Source: CAD feature listing. Evaluate the final solid. Frame: model axes, mm. A direction names the side the tool comes from. Give positions to 0.01 mm unless a question says otherwise; leave off trailing zeros. Write each loop counter-clockwise with the first axis right and the second up, starting at its lowest first coordinate (ties: lowest second). Pieces come first, ordered by that corner, then holes. Notation, with made-up numbers: M 12.25,60 L 47.25,60 A15 cw 47.25,79 Z; hole C 39.25,86 d11. An arc over 180 degrees is marked long. Answer as a JSON object with one key per item and string values. Group by question number.
Autodesk Inventor part; units mm, degrees
ref_plane "YZ Plane" through (0, 0, 0) normal (1, 0, 0) x (0, 1, 0)
ref_plane "XZ Plane" through (0, 0, 0) normal (0, 1, 0) x (-1, 0, 0)
ref_plane "XY Plane" through (0, 0, 0) normal (0, 0, 1) x (1, 0, 0)
sketch "Sketch1" plane through (0, 0, 0) normal (0, 0, 1) x (1, 0, 0)
  line L0 (-51.8104, 0) -> (51.8104, 0) construction
  line L1 (0, -35.1144) -> (0, 36.3819) construction
  line L2 (0, 0) -> (26.1682, 26.1682) construction
  line L3 (0, 0) -> (37.0074, 0) construction
  line L4 (16.8, 24.9006) -> (16.8, 21.2406)
  line L5 (16.8, 21.2406) -> (19.0203, 19.0203)
  line L6 (16.8, 24.9006) -> (0, 24.9006)
  line L7 (24.9006, 16.8) -> (21.2406, 16.8)
  line L8 (21.2406, 16.8) -> (19.0203, 19.0203)
  line L9 (24.9006, 16.8) -> (24.9006, 0)
  line L10 (0, 0) -> (-37.0074, 0) construction
  line L11 (-16.8, 24.9006) -> (-16.8, 21.2406)
  line L12 (-16.8, 21.2406) -> (-19.0203, 19.0203)
  line L13 (-16.8, 24.9006) -> (0, 24.9006)
  line L14 (-24.9006, 16.8) -> (-24.9006, 0)
  line L15 (-24.9006, 16.8) -> (-21.2406, 16.8)
  line L16 (-21.2406, 16.8) -> (-19.0203, 19.0203)
  line L17 (16.8, -24.9006) -> (16.8, -21.2406)
  line L18 (16.8, -21.2406) -> (19.0203, -19.0203)
  line L19 (16.8, -24.9006) -> (0, -24.9006)
  line L20 (24.9006, -16.8) -> (24.9006, 0)
  line L21 (24.9006, -16.8) -> (21.2406, -16.8)
  line L22 (21.2406, -16.8) -> (19.0203, -19.0203)
  line L23 (-16.8, -24.9006) -> (-16.8, -21.2406)
  line L24 (-16.8, -21.2406) -> (-19.0203, -19.0203)
  line L25 (-16.8, -24.9006) -> (0, -24.9006)
  line L26 (-24.9006, -16.8) -> (-24.9006, 0)
  line L27 (-24.9006, -16.8) -> (-21.2406, -16.8)
  line L28 (-21.2406, -16.8) -> (-19.0203, -19.0203)
  line L29 (-16.8, -16.8) -> (16.8, 16.8) construction
  line L30 (17.4242, -17.4242) -> (-16.0391, 16.0391) construction
  line L31 (-16.8, -15) -> (16.8, -15)
  line L32 (16.8, -15) -> (16.8, 15)
  line L33 (16.8, 15) -> (-16.8, 15)
  line L34 (-16.8, 15) -> (-16.8, -15)
  line L35 (-16.8, -15) -> (16.8, 15) construction
  line L36 (16.8, -15) -> (-16.8, 15) construction
  dimension "d0" = 45
  dimension "d1" = 3.14
  dimension "d2" = 3.66
  dimension "d4" = 16.8
  dimension "d16" = 33.6
  dimension "d17" = 30
extrude "Extrusion1" add sketch "Sketch1" along normal blind 8
sketch "Sketch2" plane through (-16.8, 24.9006, 0) normal (0, 1, 0) x (1, 0, 0)
  line L0 (-8.1006, 0) -> (-4.4406, 0) construction
  line L1 (-8.1006, 0) -> (-8.1006, -8) construction
  line L2 (-4.4406, -8) -> (-8.1006, -8) construction
  line L3 (-4.4406, 0) -> (-4.4406, -8) construction
  line L4 (-4.4406, 0) -> (0, 0) construction
  line L5 (-4.4406, 0) -> (-4.4406, -8) construction
  line L6 (0, -8) -> (-4.4406, -8) construction
  line L7 (0, 0) -> (0, -8) construction
  line L8 (0, 0) -> (33.6, 0) construction
  line L9 (0, 0) -> (0, -8) construction
  line L10 (33.6, -8) -> (0, -8) construction
  line L11 (33.6, 0) -> (33.6, -8) construction
  line L12 (33.6, 0) -> (38.0406, 0) construction
  line L13 (33.6, 0) -> (33.6, -8) construction
  line L14 (38.0406, -8) -> (33.6, -8) construction
  line L15 (38.0406, 0) -> (38.0406, -8) construction
  line L16 (38.0406, 0) -> (41.7006, 0) construction
  line L17 (38.0406, 0) -> (38.0406, -8) construction
  line L18 (41.7006, -8) -> (38.0406, -8) construction
  line L19 (41.7006, 0) -> (41.7006, -8) construction
  line L20 (-0.9933, -0.6346) -> (2.8461, 5.7642) construction
  ellipse E0 centre (4.1754, 7.1215) end of major axis (2.3333, 6.6563) minor radius 1.8997 (5.4585, 5.7204) -> (2.8461, 5.7642) ccw construction
  line L21 (5.4585, 5.7204) -> (9.3415, -1.2728) construction
  line L22 (9.3415, -1.2728) -> (8.4179, -1.2574) construction
  line L23 (8.4179, -1.2574) -> (4.8304, 5.2036) construction
  ellipse E1 centre (5.2675, 5.4463) end of major axis (4.7828, 5.3239) minor radius 0.4999 (4.9945, 5.8651) -> (4.8304, 5.2036) ccw construction
  ellipse E2 centre (4.1754, 7.1215) end of major axis (2.7211, 6.7542) minor radius 1.4998 (4.9945, 5.8651) -> (3.3146, 5.8932) ccw construction
  ellipse E3 centre (3.0277, 5.4838) end of major axis (3.5125, 5.6062) minor radius 0.4999 (3.4564, 5.2266) -> (3.3146, 5.8932) ccw construction
  line L24 (3.4564, 5.2266) -> (-0.3461, -1.1107) construction
  ellipse E4 centre (-1.5262, -2.0366) end of major axis (-0.0719, -1.6693) minor radius 1.4998 (-0.9933, -0.6346) -> (-0.3461, -1.1107) ccw construction
  circle A0 centre (-2.1474, -2.1474) radius 1.7
  line L25 (-4.4406, 0) -> (0, 0) construction
  line L26 (0, 0) -> (-3.5302, -3.5302) construction
  line L27 (0, 0) -> (4.9925, 0) construction
  line L28 (0, 0) -> (2, 0)
  line L29 (0, 0) -> (-1.7777, 0)
  line L30 (-1.7777, 0) -> (-2.227, -0.4493)
  line L31 (0, 0) -> (0, -3.2892)
  line L32 (0, -3.2892) -> (-0.8879, -3.2892)
  point P0 (16.8, 0)
  dimension "d8" = 3.4
  dimension "d9" = 135
extrude "Extrusion2" cut sketch "Sketch2" against normal up to surface (39.9006 mm away)
sketch "Sketch3" plane through (0, 0, 0) normal (0, 0, -1) x (-1, 0, 0)
  line L0 (16.8, 15) -> (16.8, 24.9006) construction
  line L1 (16.8, 24.9006) -> (-16.8, 24.9006) construction
  line L2 (-16.8, 24.9006) -> (-16.8, 21.2406) construction
  line L3 (-16.8, 21.2406) -> (-21.2406, 16.8) construction
  line L4 (-21.2406, 16.8) -> (-24.9006, 16.8) construction
  line L5 (-24.9006, 16.8) -> (-24.9006, -16.8) construction
  line L6 (-24.9006, -16.8) -> (-21.2406, -16.8) construction
  line L7 (-21.2406, -16.8) -> (-16.8, -21.2406) construction
  line L8 (-16.8, -21.2406) -> (-16.8, -24.9006) construction
  line L9 (-16.8, -24.9006) -> (16.8, -24.9006) construction
  line L10 (16.8, -24.9006) -> (16.8, -21.2406) construction
  line L11 (16.8, -21.2406) -> (21.2406, -16.8) construction
  line L12 (21.2406, -16.8) -> (24.9006, -16.8) construction
  line L13 (24.9006, -16.8) -> (24.9006, 16.8) construction
  line L14 (24.9006, 16.8) -> (21.2406, 16.8) construction
  line L15 (21.2406, 16.8) -> (18.5777, 19.4629) construction
  line L16 (21.2406, 16.8) -> (24.9006, 16.8) construction
  line L17 (24.9006, 16.8) -> (21.2406, 16.8)
  line L18 (18.5777, 19.4629) -> (18.5777, -15)
  line L19 (16.8, 21.2406) -> (21.2406, 16.8)
  line L20 (21.2406, 16.8) -> (16.8, 21.2406)
  line L21 (16.8, 21.2406) -> (16.8, 16.8)
  line L22 (16.8, 16.8) -> (21.2406, 16.8)
  line L23 (18.5777, 19.4629) -> (18.5777, -15)
  line L24 (18.5777, -15) -> (-16.8, -15)
  line L25 (-16.8, -15) -> (-16.8, 15)
  line L26 (-16.8, 15) -> (16.8, 15)
  point P0 (0, 0)
  point P1 (18.5777, -16.8)
extrude "Extrusion3" cut sketch "Sketch3" against normal blind 3.9
mirror "Mirror1" about plane through (0, 0, 0) normal (1, 0, 0) of "Extrusion3", "Extrusion2"
sketch "Sketch4" plane through (-16.8, -15, 8) normal (0, 1, 0) x (1, 0, 0)
  line L0 (-1.7777, 8) -> (35.3777, 8) construction
  line L1 (-1.7777, 8) -> (-2.227, 7.5507) construction
  arc A0 (-2.227, 7.5507) -> (-0.8879, 4.7108) centre (-2.1474, 5.8526) ccw construction
  line L2 (-0.8879, 4.7108) -> (0, 4.7108) construction
  line L3 (0, 4.7108) -> (0, 0) construction
  line L4 (33.6, 0) -> (0, 0) construction
  line L5 (33.6, 4.7108) -> (33.6, 0) construction
  line L6 (34.4879, 4.7108) -> (33.6, 4.7108) construction
  arc A1 (34.4879, 4.7108) -> (35.827, 7.5507) centre (35.7474, 5.8526) ccw construction
  line L7 (35.3777, 8) -> (35.827, 7.5507) construction
  circle A2 centre (35.7474, 5.8526) radius 1.7
  circle A3 centre (-2.1474, 5.8526) radius 1.7
  point P0 (16.8, 8)
extrude "Extrusion4" cut sketch "Sketch4" against normal blind 10
sketch "Sketch5" plane through (-16.8, 24.9006, 0) normal (0, 1, 0) x (1, 0, 0)
  line L0 (0, 0) -> (33.6, 0) construction
  line L1 (0, 0) -> (0, -8) construction
  line L2 (33.6, -8) -> (0, -8) construction
  line L3 (33.6, 0) -> (33.6, -8) construction
  line L4 (16.8, 0) -> (16.8, -8) construction
  line L5 (33.6, 0) -> (33.6, -8) construction
  line L6 (0, 0) -> (0, -8) construction
  line L7 (33.6, -4) -> (0, -4) construction
  line L8 (2.5, -4) -> (31.1, -4) construction
  line L9 (2.5, -5.75) -> (31.1, -5.75)
  line L10 (31.1, -2.25) -> (2.5, -2.25)
  arc A0 (2.5, -2.25) -> (2.5, -5.75) centre (2.5, -4) ccw
  arc A1 (31.1, -5.75) -> (31.1, -2.25) centre (31.1, -4) ccw
  point P0 (16.8, -4)
  dimension "d20" = 3.5
  dimension "d21" = 2.5
extrude "Extrusion5" cut sketch "Sketch5" against normal through all
sketch "Sketch6" plane through (0, 0, 8) normal (0, 0, 1) x (1, 0, 0)
  line L0 (-16.8, -15) -> (-16.8, 15)
  line L1 (-16.8, 15) -> (16.8, 15)
  line L2 (16.8, 15) -> (16.8, -15)
  line L3 (16.8, -15) -> (-16.8, -15)
  line L4 (16.8, 21.2406) -> (16.8, 24.9006)
  line L5 (16.8, 24.9006) -> (-16.8, 24.9006)
  line L6 (-16.8, 24.9006) -> (-16.8, 21.2406)
  line L7 (-16.8, 21.2406) -> (-21.2406, 16.8)
  line L8 (-21.2406, 16.8) -> (-24.9006, 16.8)
  line L9 (-24.9006, 16.8) -> (-24.9006, -16.8)
  line L10 (-24.9006, -16.8) -> (-21.2406, -16.8)
  line L11 (-21.2406, -16.8) -> (-16.8, -21.2406)
  line L12 (-16.8, -21.2406) -> (-16.8, -24.9006)
  line L13 (-16.8, -24.9006) -> (16.8, -24.9006)
  line L14 (16.8, -24.9006) -> (16.8, -21.2406)
  line L15 (16.8, -21.2406) -> (21.2406, -16.8)
  line L16 (21.2406, -16.8) -> (24.9006, -16.8)
  line L17 (24.9006, -16.8) -> (24.9006, 16.8)
  line L18 (24.9006, 16.8) -> (21.2406, 16.8)
  line L19 (21.2406, 16.8) -> (16.8, 21.2406)
  point P0 (0, 0)
extrude "Extrusion6" cut sketch "Sketch6" against normal blind 2.1
sketch "Skizze7" plane through (0, 0, 5.9) normal (0, 0, 1) x (1, 0, 0)
  line L0 (-16.8, -15) -> (16.8, -15) construction
  line L1 (-16.8, 15) -> (-16.8, -15) construction
  line L2 (16.8, 15) -> (-16.8, 15) construction
  line L3 (16.8, -15) -> (16.8, 15) construction
  line L4 (16.8, 24.9006) -> (16.8, 21.2406)
  line L5 (-16.8, 24.9006) -> (16.8, 24.9006) construction
  line L6 (-16.8, 21.2406) -> (-16.8, 24.9006)
  line L7 (-21.2406, 16.8) -> (-16.8, 21.2406)
  line L8 (-24.9006, 16.8) -> (-21.2406, 16.8)
  line L9 (-24.9006, -16.8) -> (-24.9006, 16.8) construction
  line L10 (-21.2406, -16.8) -> (-24.9006, -16.8)
  line L11 (-16.8, -21.2406) -> (-21.2406, -16.8)
  line L12 (-16.8, -24.9006) -> (-16.8, -21.2406)
  line L13 (16.8, -24.9006) -> (-16.8, -24.9006) construction
  line L14 (16.8, -21.2406) -> (16.8, -24.9006)
  line L15 (21.2406, -16.8) -> (16.8, -21.2406)
  line L16 (24.9006, -16.8) -> (21.2406, -16.8)
  line L17 (24.9006, 16.8) -> (24.9006, -16.8) construction
  line L18 (21.2406, 16.8) -> (24.9006, 16.8)
  line L19 (16.8, 21.2406) -> (21.2406, 16.8)
  line L20 (17, 25.1006) -> (17, 21.3235)
  line L21 (17, 21.3235) -> (21.3235, 17)
  line L22 (21.3235, 17) -> (25.1006, 17)
  line L23 (25.1006, 17) -> (25.1006, -17) construction
  line L24 (25.1006, -17) -> (21.3235, -17)
  line L25 (21.3235, -17) -> (17, -21.3235)
  line L26 (17, -21.3235) -> (17, -25.1006)
  line L27 (17, -25.1006) -> (-17, -25.1006) construction
  line L28 (-17, -25.1006) -> (-17, -21.3235)
  line L29 (-17, -21.3235) -> (-21.3235, -17)
  line L30 (-21.3235, -17) -> (-25.1006, -17)
  line L31 (-25.1006, -17) -> (-25.1006, 17) construction
  line L32 (-25.1006, 17) -> (-21.3235, 17)
  line L33 (-21.3235, 17) -> (-17, 21.3235)
  line L34 (-17, 21.3235) -> (-17, 25.1006)
  line L35 (-17, 25.1006) -> (17, 25.1006) construction
  line L36 (-24.9006, 16.8) -> (-24.9006, 17)
  line L37 (-16.8, 24.9006) -> (-17, 24.9006)
  line L38 (16.8, 24.9006) -> (17, 24.9006)
  line L39 (24.9006, 16.8) -> (24.9006, 17)
  line L40 (24.9006, -16.8) -> (24.9006, -17)
  line L41 (16.8, -24.9006) -> (17, -24.9006)
  line L42 (-16.8, -24.9006) -> (-17, -24.9006)
  line L43 (-24.9006, -16.8) -> (-24.9006, -17)
  point P0 (0, 0)
  dimension "d26" = 0.2
extrude "IM_offset" add sketch "Skizze7" against normal up to surface (5.9 mm away)
properties part number "20_Rect_Aperture_Insert_half_v3"
(1) Pull-direction query (Y, two-part tool) for faces 1 (the flat face through (0, 20, 2.25)), 2 (the flat face through (19.131, 19.192, 2.991)), 3 (the flat face through (0, -15, 2)), 4 (the flat face through (-21, 16.8, 2)); classes: pulls with the +Y half, pulls with the -Y half, needs draft (parallel to the pull), parting line crosses it, or undercut.
(2) Contact query for flat-ended pins moving along their axis: pin 1 Ø1.1 at (x, z) = (-22, 3) entering from -Y; pin 2 Ø3 at (y, z) = (23, 3) entering from +X; pin 3 Ø3 at (x, z) = (-3.5, 4) entering from +Y; pin 4 Ø1.8 at (y, z) = (-23.5, 1.5) entering from -X. Output: stop coordinate, or through.
(3) Ray query, L1, parallel to X at y = -15.5, z = 2.05; L2, parallel to Z at x = 0.5, y = -15.5; L3, parallel to Y at x = 16, z = 5.15. Return the intervals inside material, ascending. Write a range as [from, to].
(4) Section B-B, the plane x = -20. Return loops of the section in (y, z), plus the area to 3 significant figures.
(5) Section A-A, the plane x = -13.5. Return loops of the section in (y, z), plus the area to 3 significant figures.
(6) Access query for faces 5 (the flat face through (-18.92, -19.12, 2.17)), 6 (the flat face through (16.8, 0, 5)), 7 (the flat face through (17, 23, 3)), 8 (the flat face through (-19.05, 18.99, 1.98)). Directions: +Z, -Z, +X, -X, +Y, -Y. A direction counts if a zero-diameter tool reaches every point of the face in a straight line with its end or side. Return the directions, or none.
Reported:
{
 "1": {"face 1": "needs draft", "face 2": "pulls with the +Y half", "face 3": "undercut", "face 4": "undercut"},
 "2": {"pin 1": "stops at y = -17", "pin 2": "stops at x = 17", "pin 3": "passes through", "pin 4": "stops at x = -17"},
 "3": {"L1": "x = [-24.9, -20.64], [-17.25, 17.25], [20.64, 24.9]", "L2": "z = [0, 2.25], [5.75, 5.9]", "L3": "y = [-24.9, -15], [15, 24.9]"},
 "4": {"outline": "M -18.32,0 L 16.8,0 L 16.8,0.81 L -18.04,0.81 L -18.04,3.48 L 16.8,3.48 L 16.8,3.9 L 18.04,3.9 L 18.04,0 L 18.32,0 L 18.32,5.9 L -18.32,5.9 Z", "area": "118 mm2"},
 "5": {"outline": "M -24.9,0 L -15,0 L -15,2.25 L -24.9,2.25 Z; M -24.9,5.75 L -15,5.75 L -15,5.9 L -24.9,5.9 Z; M 15,0 L 24.9,0 L 24.9,2.25 L 15,2.25 Z; M 15,5.75 L 24.9,5.75 L 24.9,5.9 L 15,5.9 Z", "area": "47.5 mm2"},
 "6": {"face 5": "none", "face 6": "+Z, -Z", "face 7": "+Z, -Z, +X, +Y", "face 8": "-Z"}
}
